from build123d import *

# Parameters (mm, degrees)
BOSS_EXTRUDE1_DEPTH      = 6.35
BOSS_EXTRUDE1_DEPTH_BACK = 3.302
SKETCH3_R                = 4.826
CUT_EXTRUDE1_DEPTH       = 24.759524406
CUT_EXTRUDE2_DEPTH       = 33.378773911
FILLET1_R                = 2.4765


with BuildPart() as part:
    # Sketch3 → Boss-Extrude1 (new, two sides: drawn at the far end of the back side and taken through both)
    with BuildSketch(Plane.XY.offset(-BOSS_EXTRUDE1_DEPTH_BACK)):
        with BuildLine():
            Line((-12.7, 0), (12.7, 0))
            Line((12.7, 0), (12.7, 3.048))
            Line((12.7, 3.048), (7.083102209, 14.615409702))
            ThreePointArc((7.083102209, 14.615409702), (0, 19.05), (-7.083102209, 14.615409702))
            Line((-7.083102209, 14.615409702), (-12.7, 3.048))
            Line((-12.7, 3.048), (-12.7, 0))
        make_face()
        with Locations((0, 11.176)):
            Circle(SKETCH3_R, mode=Mode.SUBTRACT)
    extrude(amount=BOSS_EXTRUDE1_DEPTH + BOSS_EXTRUDE1_DEPTH_BACK)

    # Sketch4 → Cut-Extrude1 (cut, through all)
    with BuildSketch(Plane(origin=(0, 0, 0), x_dir=(1, 0, 0), z_dir=(0, 1, 0))):
        with BuildLine():
            Line((-12.7, 1.651), (-12.7, -1.651))
            Line((-12.7, -1.651), (-9.652, -1.651))
            ThreePointArc((-9.652, -1.651), (-8.001, 0), (-9.652, 1.651))
            Line((-9.652, 1.651), (-12.7, 1.651))
        make_face()
        with BuildLine():
            Line((9.652, 1.651), (12.7, 1.651))
            Line((12.7, 1.651), (12.7, -1.651))
            Line((12.7, -1.651), (9.652, -1.651))
            ThreePointArc((9.652, -1.651), (8.001, 0), (9.652, 1.651))
        make_face()
    extrude(amount=CUT_EXTRUDE1_DEPTH, mode=Mode.SUBTRACT)

    # Sketch5 → Cut-Extrude2 (cut, through all)
    with BuildSketch(Plane.ZY.offset(12.7)):
        with BuildLine():
            Line((-3.302, 19.05), (4.826, 19.05))
            Line((4.826, 19.05), (4.826, 2.286))
            ThreePointArc((4.826, 2.286), (4.602815367, 1.747184633), (4.064, 1.524))
            Line((4.064, 1.524), (-3.302, 1.524))
            Line((-3.302, 1.524), (-3.302, 19.05))
        make_face()
        with BuildLine():
            Line((4.064, 0), (6.35, 0))
            Line((6.35, 0), (6.35, 2.286))
            ThreePointArc((6.35, 2.286), (5.680446102, 0.669553898), (4.064, 0))
        make_face()
    extrude(amount=-CUT_EXTRUDE2_DEPTH, mode=Mode.SUBTRACT)

    # Fillet1
    # the kernel refuses this fillet: 2.4765 mm, written as the material it takes off along each edge
    with BuildSketch(Plane(origin=(-12.7, 7.361166479, -3.302), x_dir=(1, 0, 0), z_dir=(0, -1, 0))) as fillet1_piece_1:
        with BuildLine():
            CenterArc((2.334866591, 2.4765), FILLET1_R, 199.471220634, 70.528779366)
            Line((0, 1.651), (-0.046697332, 1.63449))
            ThreePointArc((-0.046697332, 1.63449), (-0.04953, 0.8255), (-0.04953, 0))
            Line((-0.04953, 0), (0, -0.04953))
            Line((0, -0.04953), (2.334866591, -0.04953))
            Line((2.334866591, -0.04953), (2.334866591, 0))
        make_face()
    extrude(amount=13.198332957, mode=Mode.SUBTRACT)
    with BuildSketch(Plane(origin=(12.7, -5.837166479, -3.302), x_dir=(0, 0, 1), z_dir=(0, 1, 0))) as fillet1_piece_2:
        with BuildLine():
            CenterArc((2.4765, -2.334866591), FILLET1_R, 109.471220634, 70.528779366)
            Line((0, -2.334866591), (-0.04953, -2.334866591))
            Line((-0.04953, -2.334866591), (-0.04953, 0))
            Line((-0.04953, 0), (0, 0.04953))
            ThreePointArc((0, 0.04953), (0.8255, 0.04953), (1.63449, 0.046697332))
            Line((1.63449, 0.046697332), (1.651, 0))
        make_face()
    extrude(amount=13.198332957, mode=Mode.SUBTRACT)


solid = part.part
Design review of the part built by this model. Coordinates are the model's own, in mm. A direction names the side the tool comes from. Round coordinates to 2 decimals unless told otherwise and drop trailing zeros. Loops run counter-clockwise (first coordinate to the right, second up) from the corner with the lowest first, then second, coordinate; pieces in that order, holes last. Notation, with made-up numbers: (-1, 7.5) - (49, 7.5) arc R17 cw to (49, 39.5) - close; hole circle Ø7 at (79, -10.5). An arc over 180 degrees is marked (long way). One line per question, with ' | ' between items.
1. We need section B-B, the plane y = 13.5. State the section outline as (x, z) points.
Results are:
outline: (-7.62, 4.83) - (-4.23, 4.83) - (-4.23, 6.35) - (-7.62, 6.35) - close; (4.23, 4.83) - (7.62, 4.83) - (7.62, 6.35) - (4.23, 6.35) - close
2. For L1, parallel to Z at x = 2.5, y = 3; L2, parallel to Y at x = -7.25, z = 3, list the stretches that pass through material, from the lowest coordinate up. Write a range as [from, to].
Results are:
L1: z = [4.83, 6.35] | L2: y = [0, 1.52]
3. Clearance check with flat-ended pins moving along their axes: P1, Ø2, axis at x = 6.5, y = 7.5, coming from the -Z side; P2, Ø0.8, axis at x = -11.5, y = 0.5, coming from the +Z side; P3, Ø3, axis at y = 14.5, z = 2.5, coming from the +X side; P4, Ø2, axis at x = -3.5, z = -1.5, coming from the +Y side. State where each tip first meets the part, or that it passes through.
Results are:
P1: stops at z = 4.83 | P2: stops at z = 5.88 | P3: passes through | P4: stops at y = 1.52
4. We need section D-D, the plane x = 9. State the section outline as (y, z) points, and give its area (3 significant figures).
Results are:
outline: (0, -3.3) - (1.52, -3.3) - (1.52, -1.52) - (0, -1.52) - close; (0, 1.52) - (1.52, 1.52) - (1.52, 4.06) arc R0.76 cw to (2.29, 4.83) - (10.67, 4.83) - (10.67, 6.35) - (2.29, 6.35) arc R2.29 ccw to (0, 4.06) - close | area: 23.0 mm²
5. For faces 5 (the face through (0, 1.524, 0)), 6 (the face through (-12.7, 1, 4)), 7 (the face through (11, 1, 1.651)), 8 (the face through (-11, 1, -1.651)), list the 3-axis set-ups (+Z, -Z, +X, -X, +Y, -Y) from which the entire face can be reached by the end or side of a thin tool; tool diameter is ignored.
Results are:
face 5: -Z, +X, -X, +Y | face 6: +Z, -Z, -X, +Y, -Y | face 7: +X, +Y, -Y | face 8: -X, +Y, -Y
6. We need section A-A, the plane x = 0. State the section outline as (y, z) points.
Results are:
outline: (0, -3.3) - (1.52, -3.3) - (1.52, 4.06) arc R0.76 cw to (2.29, 4.83) - (6.35, 4.83) - (6.35, 6.35) - (2.29, 6.35) arc R2.29 ccw to (0, 4.06) - close; (16, 4.83) - (19.05, 4.83) - (19.05, 6.35) - (16, 6.35) - close
7. Draft analysis for pull direction Z (two halves, no side actions). For faces 1 (the face through (12.7, 1, 4)), 2 (the face through (0, 1, -3.302)), 3 (the face through (11, 1, -1.651)), 4 (the face through (-11, 1, 1.651)), state which applies: released by +Z, released by -Z, zero draft, split by the parting line, or undercut.
Results are:
face 1: zero draft | face 2: released by -Z | face 3: undercut | face 4: undercut
8. We need section C-C, the plane z = 2.75. State the section outline as (x, y) points, and give its area (3 significant figures).
Results are:
outline: (-12.7, 0) - (12.7, 0) - (12.7, 1.52) - (-12.7, 1.52) - close | area: 38.7 mm²
